Design review of the part built by this model. Coordinates are the model's own, in mm. A direction names the side the tool comes from. Coordinates: 2 decimals unless noted, no trailing zeros. Loops run counter-clockwise (first coordinate to the right, second up) from the corner with the lowest first, then second, coordinate; pieces in that order, holes last.
Autodesk Inventor part; units mm, degrees
ref_plane "YZ Plane" through (0, 0, 0) normal (1, 0, 0) x (0, 1, 0)
ref_plane "XZ Plane" through (0, 0, 0) normal (0, 1, 0) x (-1, 0, 0)
ref_plane "XY Plane" through (0, 0, 0) normal (0, 0, 1) x (1, 0, 0)
sketch "Sketch1" plane through (0, 0, 0) normal (1, 0, 0) x (0, 1, 0)
  point P0 (0, 0)
sketch "Sketch2" plane through (0, 0, 0) normal (1, 0, 0) x (0, 1, 0)
  line L0 (0, 0) -> (0, -431.8)
  line L1 (0, -431.8) -> (88.9, -431.8)
  line L2 (88.9, -431.8) -> (88.9, -88.9)
  line L3 (88.9, -88.9) -> (749.3, -88.9)
  line L4 (749.3, -88.9) -> (749.3, -431.8)
  line L5 (749.3, -431.8) -> (838.2, -431.8)
  line L6 (838.2, -431.8) -> (838.2, 0)
  line L7 (838.2, 0) -> (0, 0)
  dimension "d0" = 660.4
  dimension "d1" = 342.9
  dimension "d2" = 342.9
  dimension "d3" = 88.9
  dimension "d4" = 88.9
  dimension "d5" = 88.9
extrude "Extrusion1" add sketch "Sketch2" along normal blind 127
fillet "Fillet1" radius 25.4 14 edges at (127, 419.1, 0) (0, 419.1, 0) (63.5, 838.2, 0) (127, 838.2, -215.9) (0, 838.2, -215.9) (63.5, 0, 0) (127, 0, -215.9) (127, 44.45, -431.8) (127, 793.75, -431.8) (63.5, 838.2, -431.8) (0, 793.75, -431.8) (0, 0, -215.9) (0, 44.45, -431.8) (63.5, 0, -431.8)
sketch "Sketch7" plane through (0, 88.9, -88.9) normal (0, 0, -1) x (-1, 0, 0)
  line L0 (-127, 0) -> (-127, 660.4)
  line L1 (-127, 0) -> (-127, 660.4)
  line L2 (-127, 660.4) -> (-127, 647.7)
  line L3 (-127, -63.5) -> (-127, 723.9)
  line L4 (-127, 0) -> (-127, 12.7)
  line L5 (-127, 12.7) -> (-127, 139.7)
  line L6 (-127, 139.7) -> (-127, 266.7)
  line L7 (-127, 266.7) -> (-127, 393.7)
  line L8 (-127, 393.7) -> (-127, 520.7)
  line L9 (-127, 520.7) -> (-127, 647.7)
  line L10 (-127, 330.2) -> (0, 330.2)
  line L11 (-127, 520.7) -> (0, 520.7)
  line L12 (0, 0) -> (0, 660.4)
  line L13 (-127, 139.7) -> (0, 139.7)
  line L14 (-127, 139.7) -> (-117.475, 139.7)
  line L15 (-127, 330.2) -> (-117.475, 330.2)
  line L16 (-127, 520.7) -> (-117.475, 520.7)
  line L17 (-117.475, 139.7) -> (-117.475, 165.1)
  line L18 (-117.475, 139.7) -> (-117.475, 114.3)
  line L19 (-117.475, 330.2) -> (-117.475, 304.8)
  line L20 (-117.475, 304.8) -> (-117.475, 355.6)
  line L21 (-117.475, 520.7) -> (-117.475, 495.3)
  line L22 (-117.475, 495.3) -> (-117.475, 546.1)
  circle A0 centre (-117.475, 114.3) radius 2.54
  circle A1 centre (-117.475, 165.1) radius 2.54
  circle A2 centre (-117.475, 304.8) radius 2.54
  circle A3 centre (-117.475, 355.6) radius 2.54
  circle A4 centre (-117.475, 495.3) radius 2.54
  circle A5 centre (-117.475, 546.1) radius 2.54
  line L23 (0, 139.7) -> (-9.525, 139.7)
  line L24 (-9.525, 139.7) -> (-9.525, 114.3)
  line L25 (-9.525, 114.3) -> (-9.525, 165.1)
  line L26 (-9.525, 304.8) -> (-9.525, 330.2)
  line L27 (-9.525, 330.2) -> (-9.525, 355.6)
  line L28 (-9.525, 495.3) -> (-9.525, 520.7)
  line L29 (-9.525, 520.7) -> (-9.525, 546.1)
  circle A6 centre (-9.525, 114.3) radius 2.54
  circle A7 centre (-9.525, 165.1) radius 2.54
  circle A8 centre (-9.525, 304.8) radius 2.54
  circle A9 centre (-9.525, 355.6) radius 2.54
  circle A10 centre (-9.525, 495.3) radius 2.54
  circle A11 centre (-9.525, 546.1) radius 2.54
  point P0 (0, -88.9)
  dimension "d52" = 12.7
  dimension "d53" = 12.7
  dimension "d54" = 127
  dimension "d55" = 127
  dimension "d56" = 127
  dimension "d57" = 127
  dimension "d58" = 9.525
  dimension "d59" = 25.4
  dimension "d60" = 25.4
  dimension "d61" = 25.4
  dimension "d62" = 50.8
  dimension "d63" = 25.4
  dimension "d64" = 50.8
  dimension "d65" = 5.08
  dimension "d66" = 9.525
extrude "Extrusion7" cut sketch "Sketch7" against normal blind 25.4 contours A5 | A11 | A6 | A0 | A1 | A7 | A8 | A2 | A3 | A9 | A10 | A4
properties part number "Bumper"
Q1. The part is to be moulded in two halves that separate along Y. For faces 3 (the flat face through (63, 414, -88.9)), 4 (the cylindrical face through (7.64, 781.49, -424.56)), 5 (the cylindrical face through (119.76, 7.64, -218.57)), say which applies: pulls with the +Y half, pulls with the -Y half, needs draft (parallel to the pull), parting line crosses it, or undercut.
Q2. Take a section at B-B, the plane y = 149. Write out the cut boundary in (x, z).
Q3. Take a section at C-C, the plane x = 68.5. Write out the cut boundary in (y, z).
Q4. For line 1 (X direction, y = 444.5, z = -79) (3 decimals); line 2 (Y direction, x = 34.5, z = -223); line 3 (Y direction, x = 23, z = -162), list the stretches that pass through material, from the lowest coordinate up.
Q5. Take a section at A-A, the plane z = -237.5. Write out the cut boundary in (x, y).
Q6. Clearance check with flat-ended pins moving along their axes: pin 1 Ø4 at (x, y) = (9, 394.5) entering from -Z; pin 2 Ø4 at (x, y) = (117.475, 635) entering from -Z; pin 3 Ø6 at (x, y) = (117.475, 254) entering from +Z. State where each tip first meets the part, or that it passes through.
Q7. Machinability: for faces 1 (the flat face through (63, 749.3, -258)), 2 (the flat face through (63, 57, -431.8)), which of the approach directions +Z, -Z, +X, -X, +Y, -Y give a long, thin tool a straight path to every point of the face, cutting with its end or side? Answer none if there is none.
Entries:
1. face 3: undercut
1. face 4: needs draft
1. face 5: pulls with the -Y half
2. outline: (0, -88.9) - (127, -88.9) - (127, -25.4) arc R25.4 ccw to (101.6, 0) - (25.4, 0) arc R25.4 ccw to (0, -25.4) - close
3. outline: (0, -406.4) arc R25.4 ccw to (25.4, -431.8) - (88.9, -431.8) - (88.9, -88.9) - (749.3, -88.9) - (749.3, -431.8) - (812.8, -431.8) arc R25.4 ccw to (838.2, -406.4) - (838.2, -25.4) arc R25.4 ccw to (812.8, 0) - (25.4, 0) arc R25.4 ccw to (0, -25.4) - close
4. line 1: x = 0 to 6.985, 12.065 to 114.935, 120.015 to 127
4. line 2: y = 0 to 88.9, 749.3 to 838.2
4. line 3: y = 0.11 to 88.9, 749.3 to 838.09
5. outline: (0, 25.4) arc R25.4 ccw to (25.4, 0) - (101.6, 0) arc R25.4 ccw to (127, 25.4) - (127, 88.9) - (0, 88.9) - close; (0, 749.3) - (127, 749.3) - (127, 812.8) arc R25.4 ccw to (101.6, 838.2) - (25.4, 838.2) arc R25.4 ccw to (0, 812.8) - close
6. pin 1: stops at z = -88.9
6. pin 2: stops at z = -63.5
6. pin 3: stops at z = -3.5
7. face 1: -Z, +X, -X
7. face 2: -Z, +X, -X, +Y, -Y
